Build history of the part. All positions in model axes, mm. Face numbers are marked on the shaded views. A direction names the side the tool comes from. Round coordinates to 2 decimals unless told otherwise and drop trailing zeros. Write each loop counter-clockwise with the first axis right and the second up, starting at its lowest first coordinate (ties: lowest second). Pieces come first, ordered by that corner, then holes. Notation, with made-up numbers: (20.25, -17.5) -> (61.25, -17.5) arc R24 cw to (61.25, 16.5) -> close; hole circle Ø10 at (79.5, 44). An arc over 180 degrees is marked (long way). Answer in a Markdown table with one row per item.
Autodesk Inventor part; units mm, degrees
ref_plane "YZ Plane" through (0, 0, 0) normal (1, 0, 0) x (0, 1, 0)
ref_plane "XZ Plane" through (0, 0, 0) normal (0, 1, 0) x (-1, 0, 0)
ref_plane "XY Plane" through (0, 0, 0) normal (0, 0, 1) x (1, 0, 0)
sketch "Skizze1" plane through (0, 0, 0) normal (0, 0, 1) x (1, 0, 0)
  line L0 (-8.4, 0) -> (8.4, 0)
  line L1 (0, -7) -> (0, 7)
  line L2 (-6, 5) -> (6, 5)
  line L3 (6, 5) -> (6, -5)
  line L4 (6, -5) -> (-6, -5)
  line L5 (-6, -5) -> (-6, 5)
  point P0 (0, 0)
  dimension "d0" = 10
  dimension "d1" = 12
extrude "Extrusion1" add sketch "Skizze1" along normal blind 26
sketch "Skizze2" plane through (0, 0, 26) normal (0, 0, 1) x (1, 0, 0)
  circle A0 centre (0, 0) radius 2
  dimension "d4" = 4
extrude "Extrusion2" add sketch "Skizze2" along normal blind 0.65
sketch "Skizze3" plane through (0, 0, 26) normal (0, 0, 1) x (1, 0, 0)
  circle A0 centre (0, 0) radius 2
  circle A1 centre (0, 0) radius 1.5
  dimension "d7" = 3
extrude "Extrusion3" add sketch "Skizze3" along normal blind 4.5 contours A1
sketch "Skizze4" plane through (0, 0, 26) normal (0, 0, 1) x (1, 0, 0)
  line L0 (-8.4, 0) -> (8.4, 0)
  line L1 (0, -7) -> (0, 7)
  line L2 (-4, 3) -> (4, 3)
  line L3 (4, 3) -> (4, -3)
  line L4 (4, -3) -> (-4, -3)
  line L5 (-4, -3) -> (-4, 3)
  dimension "d10" = 6
  dimension "d11" = 8
hole "Bohrung1" at (-4, -3, 26) at (4, 3, 26) at (-4, -3, 26) at (4, 3, 26) direction (0, 0, -1) diameter 1.4 depth 8 tip angle 118 countersink diameter 2.5 countersink angle 90
sketch "Skizze5" plane through (0, 0, 26) normal (0, 0, 1) x (1, 0, 0)
  line L0 (-8.4, 0) -> (8.4, 0)
  line L1 (0, -7) -> (0, 7)
  point P0 (-4.5, 0)
  point P1 (4.5, 0)
  dimension "d19" = 9
hole "Bohrung2" at (-4.5, 0, 26) at (4.5, 0, 26) direction (0, 0, -1) diameter 1.221 depth 8 tip angle 118
sketch "Skizze6" plane through (0, 0, 0) normal (0, 0, -1) x (-1, 0, 0)
  circle A0 centre (0, 0) radius 0.5
  dimension "d27" = 1
extrude "Extrusion4" add sketch "Skizze6" along normal blind 8
sketch "Skizze8" plane through (0, 0, 0) normal (0, 0, -1) x (-1, 0, 0)
  circle A0 centre (0, 0) radius 0.5
  line L0 (6, 5) -> (-6, 5)
  line L1 (-6, 5) -> (-6, -5)
  line L2 (-6, -5) -> (6, -5)
  line L3 (6, -5) -> (6, 5)
  arc A1 (-3.2253, 5) -> (-3.2253, -5) centre (0, 0) ccw
  arc A2 (3.2253, -5) -> (3.2253, 5) centre (0, 0) ccw
  dimension "d38" = 5.95
  dimension "d39" = 5.95
extrude "Extrusion6" cut sketch "Skizze8" against normal blind 16 contours L3 L2 A2 L0 | A1 L2 L1 L0
sketch "Skizze9" plane through (0, 0, 30.5) normal (0, 0, 1) x (1, 0, 0)
  circle A0 centre (0, 0) radius 1.5
  line L0 (-1.118, 1) -> (1.118, 1)
  dimension "d42" = 1
extrude "Extrusion7" cut sketch "Skizze9" against normal up to surface (3.85 mm away) contours L0 A0 picked at (-0.0599, 1.1631)
properties part number "Motor XDRIVE GM12F"
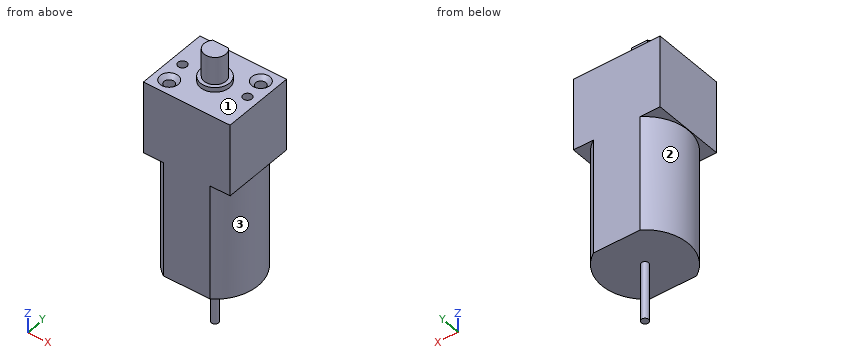
Q1. Drop flat-ended pins along their axis: P1, Ø2, axis at x = -4, y = -3, coming from the -Z side; P2, Ø0.7, axis at x = 4.5, y = 0, coming from the +Z side; P3, Ø1.5, axis at x = 4, z = 0, coming from the -Y side; P4, Ø6, axis at x = -2, y = 0.5, coming from the -Z side. Give the stop position or say it passes through.
A:
| item | result |
|---|---|
| P1 | z = 0 |
| P2 | z = 17.84 |
| P3 | y = -4.98 |
| P4 | z = -8 |
Q2. Which spindle directions (+Z, -Z, +X, -X, +Y, -Y) get a long thin tool onto all of the face, cutting with end or side? Do the marked faces 1, 2 and 3. Say none if no direction does.
A:
| item | result |
|---|---|
| face 1 | +Z |
| face 2 | -Z, -X |
| face 3 | -Z, +X |
Q3. Saw through at B-B on x = 0. Write the cut outline in (y, z).
A:
| item | result |
|---|---|
| outline | (-5, 0) -> (-0.5, 0) -> (-0.5, -8) -> (0.5, -8) -> (0.5, 0) -> (5, 0) -> (5, 26) -> (2, 26) -> (2, 26.65) -> (1, 26.65) -> (1, 30.5) -> (-1.5, 30.5) -> (-1.5, 26.65) -> (-2, 26.65) -> (-2, 26) -> (-5, 26) -> close |
Q4. Saw through at D-D on z = -3.5. Write the cut outline in (x, y).
A:
| item | result |
|---|---|
| outline | circle Ø1 at (0, 0) |
Q5. Saw through at A-A on z = 23.5. Write the cut outline in (x, y).
A:
| item | result |
|---|---|
| outline | (-6, -5) -> (6, -5) -> (6, 5) -> (-6, 5) -> close; hole circle Ø1.22 at (-4.5, 0); hole circle Ø1.4 at (-4, -3); hole circle Ø1.4 at (4, 3); hole circle Ø1.22 at (4.5, 0) |
Q6. Wall check: line 1 (X direction, y = 0, z = 20.5); line 2 (X direction, y = 0.5, z = 24.5); line 3 (Y direction, x = 4.5, z = 20.5). Give the ranges that are in metal, low to high. Write a range as [from, to].
A:
| item | result |
|---|---|
| line 1 | [-6, -5.11], [-3.89, 3.89], [5.11, 6] |
| line 2 | [-6, -4.85], [-4.15, 4.15], [4.85, 6] |
| line 3 | [-5, -0.61], [0.61, 2.51], [3.49, 5] |
Q7. Saw through at C-C on z = 8.5. Write the cut outline in (x, y), plus the area to 3 significant figures.
A:
| item | result |
|---|---|
| outline | (-3.23, -5) -> (3.23, -5) arc R5.95 ccw to (3.23, 5) -> (-3.23, 5) arc R5.95 ccw to start |
| area | 103 mm² |
